```python
from build123d import *

# Parameters (mm, degrees)
F0_W     = 2032
F0_H     = 203.2
F1_DEPTH = 25.4


with BuildPart() as f1:
    # F0 (on Front) → F1 (new body)
    with BuildSketch(Plane.XZ):
        with Locations((-92.64186, 36.177602)):
            Rectangle(F0_W, F0_H)
        with BuildLine():
            ThreePointArc((-554.92186, -27.322398), (-558.641603, -36.302654), (-567.62186, -40.022398))
            Line((-567.62186, -40.022398), (-755.123796, -40.022398))
            ThreePointArc((-755.123796, -40.022398), (-767.484058, -30.24026), (-760.803409, -15.963173))
            Line((-760.803409, -15.963173), (-573.301472, 77.787796))
            ThreePointArc((-573.301472, 77.787796), (-560.945074, 77.231836), (-554.92186, 66.42857))
            Line((-554.92186, 66.42857), (-554.92186, -27.322398))
        make_face(mode=Mode.SUBTRACT)
        with BuildLine():
            Line((-930.830474, -8.218414), (-930.84186, -8.601821))
            Line((-930.84186, -8.601821), (-930.84186, 74.277602))
            ThreePointArc((-930.84186, 74.277602), (-927.122116, 83.257858), (-918.14186, 86.977602))
            Line((-918.14186, 86.977602), (-736.012165, 86.977602))
            ThreePointArc((-736.012165, 86.977602), (-723.594962, 76.942764), (-730.800533, 62.696199))
            Line((-730.800533, 62.696199), (-912.930228, -19.262164))
            ThreePointArc((-912.930228, -19.262164), (-924.810249, -18.48921), (-930.830474, -8.218414))
        make_face(mode=Mode.SUBTRACT)
        with BuildLine():
            Line((-493.96186, -27.322398), (-493.96186, 66.42857))
            ThreePointArc((-493.96186, 66.42857), (-487.938645, 77.231836), (-475.582247, 77.787796))
            Line((-475.582247, 77.787796), (-288.08031, -15.963173))
            ThreePointArc((-288.08031, -15.963173), (-281.399661, -30.24026), (-293.759923, -40.022398))
            Line((-293.759923, -40.022398), (-481.26186, -40.022398))
            ThreePointArc((-481.26186, -40.022398), (-490.242116, -36.302654), (-493.96186, -27.322398))
        make_face(mode=Mode.SUBTRACT)
        with BuildLine():
            Line((-118.04186, 74.277602), (-118.04186, -8.601821))
            Line((-118.04186, -8.601821), (-118.053245, -8.218414))
            ThreePointArc((-118.053245, -8.218414), (-124.07347, -18.48921), (-135.953491, -19.262164))
            Line((-135.953491, -19.262164), (-318.083186, 62.696199))
            ThreePointArc((-318.083186, 62.696199), (-325.288757, 76.942764), (-312.871555, 86.977602))
            Line((-312.871555, 86.977602), (-130.74186, 86.977602))
            ThreePointArc((-130.74186, 86.977602), (-121.761603, 83.257858), (-118.04186, 74.277602))
        make_face(mode=Mode.SUBTRACT)
        with BuildLine():
            Line((-67.24186, -8.601821), (-67.24186, 74.277602))
            ThreePointArc((-67.24186, 74.277602), (-63.522116, 83.257858), (-54.54186, 86.977602))
            Line((-54.54186, 86.977602), (127.587835, 86.977602))
            ThreePointArc((127.587835, 86.977602), (140.005038, 76.942764), (132.799467, 62.696199))
            Line((132.799467, 62.696199), (-49.330228, -19.262164))
            ThreePointArc((-49.330228, -19.262164), (-61.210249, -18.48921), (-67.230474, -8.218414))
            Line((-67.230474, -8.218414), (-67.24186, -8.601821))
        make_face(mode=Mode.SUBTRACT)
        with BuildLine():
            ThreePointArc((290.298528, 77.787796), (302.654926, 77.231836), (308.67814, 66.42857))
            Line((308.67814, 66.42857), (308.67814, -27.322398))
            ThreePointArc((308.67814, -27.322398), (304.958397, -36.302654), (295.97814, -40.022398))
            Line((295.97814, -40.022398), (108.476204, -40.022398))
            ThreePointArc((108.476204, -40.022398), (96.115942, -30.24026), (102.796591, -15.963173))
            Line((102.796591, -15.963173), (290.298528, 77.787796))
        make_face(mode=Mode.SUBTRACT)
        with BuildLine():
            Line((388.017753, 77.787796), (575.51969, -15.963173))
            ThreePointArc((575.51969, -15.963173), (582.200339, -30.24026), (569.840077, -40.022398))
            Line((569.840077, -40.022398), (382.33814, -40.022398))
            ThreePointArc((382.33814, -40.022398), (373.357884, -36.302654), (369.63814, -27.322398))
            Line((369.63814, -27.322398), (369.63814, 66.42857))
            ThreePointArc((369.63814, 66.42857), (375.661355, 77.231836), (388.017753, 77.787796))
        make_face(mode=Mode.SUBTRACT)
        with BuildLine():
            Line((550.728445, 86.977602), (732.85814, 86.977602))
            ThreePointArc((732.85814, 86.977602), (741.838397, 83.257858), (745.55814, 74.277602))
            Line((745.55814, 74.277602), (745.55814, -8.601821))
            Line((745.55814, -8.601821), (745.546755, -8.218414))
            ThreePointArc((745.546755, -8.218414), (739.52653, -18.48921), (727.646509, -19.262164))
            Line((727.646509, -19.262164), (545.516814, 62.696199))
            ThreePointArc((545.516814, 62.696199), (538.311243, 76.942764), (550.728445, 86.977602))
        make_face(mode=Mode.SUBTRACT)
    extrude(amount=F1_DEPTH)


solid = f1.part
```
Verification items for the finished model (mm, model axes). A direction names the side the tool comes from. Coordinates: 2 decimals unless noted, no trailing zeros. Loops run counter-clockwise (first coordinate to the right, second up) from the corner with the lowest first, then second, coordinate; pieces in that order, holes last. Notation, with made-up numbers: (-19, -22) - (31, -22) arc R20 cw to (31, 13) - close; hole circle Ø7 at (67.25, 32.5). An arc over 180 degrees is marked (long way). Put each result on its own line as item: value.
Item 1: Scan lines: line 1 along Z through (x, y) = (382, -0.75); line 2 along X through (y, z) = (-23, 81); line 3 along X through (y, z) = (-5.5, -33.5). Record each from-to range of solid material in increasing order.
Conclusion:
line 1: z = -65.42 to -40.02, 79.12 to 137.78
line 2: x = -1108.64 to -928.92, -725.24 to -323.65, -119.97 to -65.32, 138.36 to 539.95, 743.63 to 923.36
line 3: x = -1108.64 to -766.22, -556.53 to -492.36, -282.66 to 97.38, 307.07 to 371.24, 580.94 to 923.36
Item 2: Draft check along Z on faces 3 (the face through (-107, -25.4, 38)), 4 (the face through (-820.59, -12.52, 22.29)). Enter one of: pulls with the +Z half, pulls with the -Z half, needs draft (parallel to the pull), parting line crosses it, or undercut.
Conclusion:
face 3: needs draft
face 4: undercut
Item 3: Section check B-B (y = -5.75). Give the number of separate pieces and of enclosed holes in the cut face, then the cut area to 3 significant figures.
Conclusion:
separate pieces: 1
enclosed holes: 8
area: 295,000 mm2
Item 4: Gauge pin test, flat end, axial feed: pin 1 Ø4 at (x, z) = (234.5, 106.5) entering from +Y. Record the tip position at first contact, or that the pin passes through.
Conclusion:
pin 1: stops at y = 0
Item 5: Set-up check for faces 1 (the face through (480.456, -12.522, 31.569)), 2 (the face through (-107, 0, 38)): record each of +Z, -Z, +X, -X, +Y, -Y from which the full face is reachable in a straight line by a thin tool's end or side.
Conclusion:
face 1: +Y, -Y
face 2: +Z, -Z, +X, -X, +Y
Item 6: Section check A-A (x = -368). Enter the section's corners in (y, z).
Conclusion:
outline: (-25.4, -65.42) - (0, -65.42) - (0, -40.02) - (-25.4, -40.02) - close; (-25.4, 24) - (0, 24) - (0, 137.78) - (-25.4, 137.78) - close
Item 7: Section check C-C (x = 74.5). Enter the section's corners in (y, z).
Conclusion:
outline: (-25.4, -65.42) - (0, -65.42) - (0, 36.46) - (-25.4, 36.46) - close; (-25.4, 86.98) - (0, 86.98) - (0, 137.78) - (-25.4, 137.78) - close
